Could you check a few things on this drawing? It's one solid part, dimensions in mm from its lowest x, y, z. A direction names the side the tool comes from. Coordinates: 2 decimals unless noted, no trailing zeros. Order: outer loops, then holes, each group sorted by start corner. A loop starts at its lowest first (then second) coordinate and runs counter-clockwise, first axis right, second up. Notation, with made-up numbers: M 11,69.5 L 22,69.5 A14 cw 22,77.5 Z; hole C 69,21 d4. An arc over 180 degrees is marked long. Write item = value, one per line. Start each with the question number.
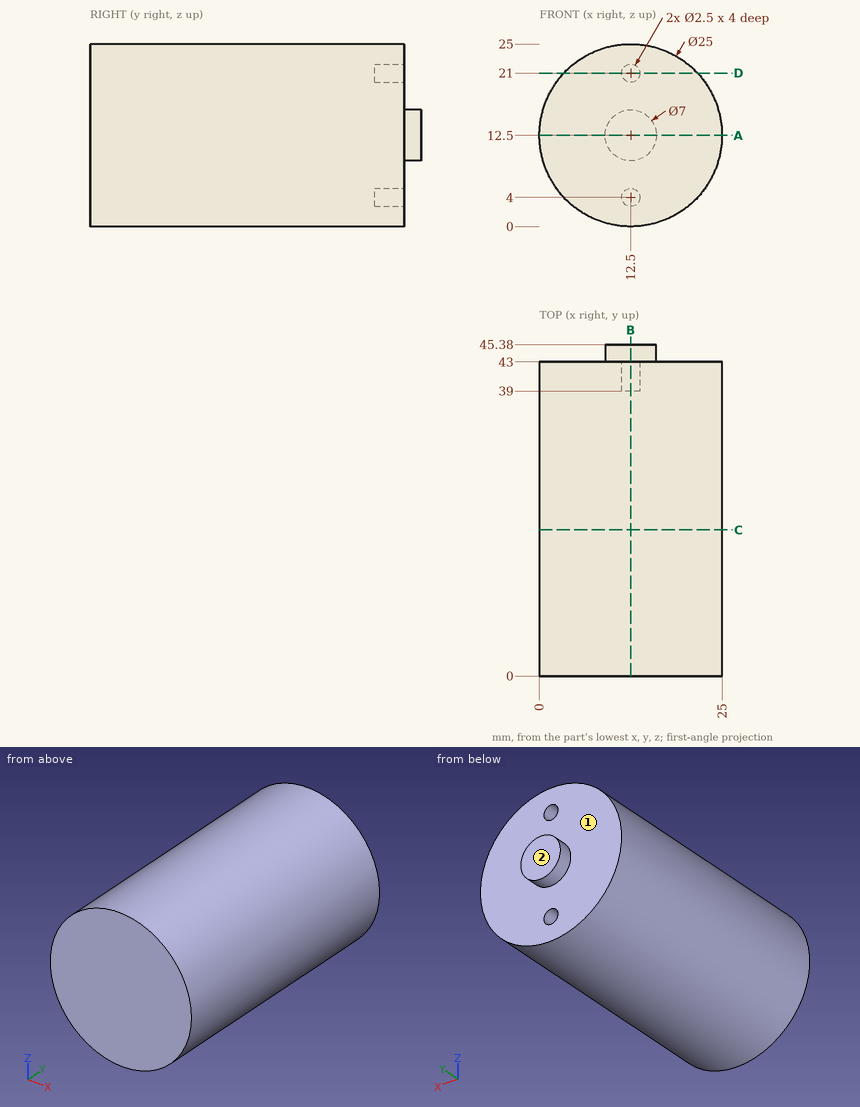
(1) Will these pins go through, and if not, where does the flat tip stop? P1, Ø1.2, axis at x = 12, z = 21, coming from the +Y side; P2, Ø3, axis at x = 12.5, z = 21, coming from the -Y side; P3, Ø3, axis at x = 12, z = 3.5, coming from the +Y side; P4, Ø8, axis at y = 10.5, z = 19.5, coming from the +X side.
(2) Imagine slicing it at D-D on z = 21. List the corners of the cut face in (x, y) for me, plus the area to 3 significant figures.
(3) Imagine slicing it at A-A on z = 12.5. List the corners of the cut face in (x, y) for me, plus the area to 3 significant figures.
(4) Imagine slicing it at C-C on y = 20. List the corners of the cut face in (x, z) for me.
(5) Please list where these lines run through material, in increasing order: probe 1 along Z at (x, y) = (12.5, 40.95); probe 2 along Y at (x, z) = (8, 1.5); probe 3 along X at (y, z) = (40.8, 21). Write a range as from..to.
(6) For the marked faces 1 and 2, which set-ups out of +Z, -Z, +X, -X, +Y, -Y let a thin tool reach every point of the face, with its end or its side?
(7) Imagine slicing it at B-B on x = 12.5. List the corners of the cut face in (y, z) for me, plus the area to 3 significant figures.
Response:
q1.P1 = 39
q1.P2 = 0
q1.P3 = 43
q1.P4 = 24.63
q2.outline = M 3.33,0 L 21.67,0 L 21.67,43 L 13.75,43 L 13.75,39 L 11.25,39 L 11.25,43 L 3.33,43 Z
q2.area = 778 mm2
q3.outline = M 0,0 L 25,0 L 25,43 L 16,43 L 16,45.38 L 9,45.38 L 9,43 L 0,43 Z
q3.area = 1,090 mm2
q4.outline = C 12.5,12.5 d25
q5.probe_1 = 0..2.75, 5.25..19.75, 22.25..25
q5.probe_2 = 0..43
q5.probe_3 = 3.33..11.25, 13.75..21.67
q6.face_1 = +Y
q6.face_2 = +Z, -Z, +X, -X, +Y
q7.outline = M 0,0 L 43,0 L 43,2.75 L 39,2.75 L 39,5.25 L 43,5.25 L 43,9 L 45.38,9 L 45.38,16 L 43,16 L 43,19.75 L 39,19.75 L 39,22.25 L 43,22.25 L 43,25 L 0,25 Z
q7.area = 1,070 mm2
